```python
from build123d import *

# Parameters (mm, degrees)
F0_W           = 190
F0_H           = 30
F1_DEPTH       = 16
F3_D           = 10
F4_D           = 5
F4_CSINK_D     = 10
F4_CSINK_ANGLE = 82


with BuildPart() as f1:
    # F0 (on Front) → F1 (new body)
    with BuildSketch(Plane.XZ):
        with Locations((95, -15)):
            Rectangle(F0_W, F0_H)
    extrude(amount=F1_DEPTH)

    # F3 (through all)
    with Locations(Plane.XZ.offset(16)):
        with Locations((40, -15), (150, -15)):
            Hole(F3_D / 2)

    # F4 (through all)
    with Locations(Plane.XZ.offset(16)):
        with Locations((10, -15), (95, -15), (180, -15)):
            CounterSinkHole(F4_D / 2, F4_CSINK_D / 2, counter_sink_angle=F4_CSINK_ANGLE)


solid = f1.part
```
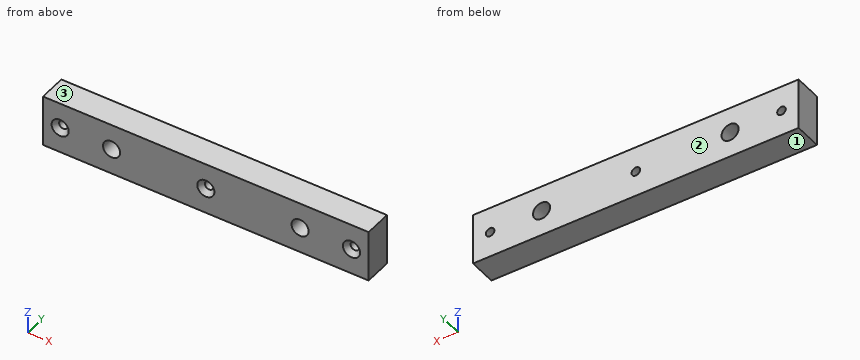
Source: CAD feature listing. Evaluate the final solid. Frame: model axes, mm. Face numbers are marked on the shaded views. Round coordinates to 2 decimals unless told otherwise and drop trailing zeros. Write each loop counter-clockwise with the first axis right and the second up, starting at its lowest first coordinate (ties: lowest second). Pieces come first, ordered by that corner, then holes. Notation, with made-up numbers: M 80,-12 L 121,-12 A8 ccw 121,-2 Z; hole C 5.25,-20 d8. An arc over 180 degrees is marked long. Answer as a JSON object with one key per item and string values. Group by question number.
(1) Section query A-A on x = 95. Output: boundary loops of the cut face in (y, z), then the cut area to 3 significant figures.
(2) Section query B-B on z = -15. State how many separate pieces and enclosed holes the cut face has, then the cut area to 3 significant figures.
(3) Section query C-C on y = -7. Output: boundary loops of the cut face in (x, z), then the cut area to 3 significant figures.
(4) Ray query, line 1 (Z direction, x = 150, y = -12.5); line 2 (Z direction, x = 180, y = -2.75); line 3 (X direction, y = -5.5, z = -16.5). Return the intervals inside material, ascending. Write a range as [from, to].
(5) Mould query, pull axis Z, two halves, no side actions, for the marked faces 1, 2 and 3. Classes: +Z half, -Z half, draft (parallel to the pull), parting line (faces both ways), or undercut.
(6) Section query D-D on x = 40. Output: boundary loops of the cut face in (y, z).
Computed values:
{
 "1": {"outline": "M -16,-30 L 0,-30 L 0,-17.5 L -13.12,-17.5 L -16,-20 Z; M -16,-10 L -13.12,-12.5 L 0,-12.5 L 0,0 L -16,0 Z", "area": "393 mm^2"},
 "2": {"separate pieces": "6", "enclosed holes": "0", "area": "2,460 mm^2"},
 "3": {"outline": "M 0,-30 L 190,-30 L 190,0 L 0,0 Z; hole C 10,-15 d5; hole C 40,-15 d10; hole C 95,-15 d5; hole C 150,-15 d10; hole C 180,-15 d5", "area": "5,480 mm^2"},
 "4": {"line 1": "[-30, -20], [-10, 0]", "line 2": "[-30, -17.5], [-12.5, 0]", "line 3": "[0, 8], [12, 35.23], [44.77, 93], [97, 145.23], [154.77, 178], [182, 190]"},
 "5": {"face 1": "-Z half", "face 2": "draft", "face 3": "+Z half"},
 "6": {"outline": "M -16,-30 L 0,-30 L 0,-20 L -16,-20 Z; M -16,-10 L 0,-10 L 0,0 L -16,0 Z"}
}
